Can you work these out from the model? Positions are in its coordinate system, mm. A direction names the side the tool comes from. Round coordinates to 2 decimals unless told otherwise and drop trailing zeros. Write each loop counter-clockwise with the first axis right and the second up, starting at its lowest first coordinate (ties: lowest second). Pieces come first, ordered by that corner, then holes. Notation, with made-up numbers: (60, -26.5) - (73, -26.5) arc R27 ccw to (73, -5.5) - close; hole circle Ø11 at (-31.5, 24). An arc over 180 degrees is marked (long way). One line per item, written item: value. Start each with the question number.
(1) I'm going to push flat-ended pins straight in: pin 1 Ø4 at (x, z) = (21.5, -6.5) entering from -Y; pin 2 Ø8 at (y, z) = (-39, -13) entering from -X; pin 3 Ø5 at (y, z) = (-66, -8.5) entering from -X; pin 4 Ø23 at (x, y) = (0, 115.25) entering from +Z. Where does each tip first touch, or does it pass through?
(2) Thinking about a two-plate mould opening in Y: for faces 1 (the face through (64, -64, -20)), 2 (the face through (-1, 17, -12)), 3 (the face through (-32.08, -144.48, -9.86)), which applies, +Y half, -Y half, draft (parallel to the pull), parting line (faces both ways), or undercut?
(3) I want a section at A-A on y = 0. List the corners of the cut face in (x, z) for me.
(4) I want a section at C-C on x = -105. List the corners of the cut face in (y, z) for me, plus the area to 3 significant figures.
(5) On a 3-axis mill with a long thin cutter (end or side, diameter ignored), from which of +Z, -Z, +X, -X, +Y, -Y can I reach the whole of each face in a straight line? I mean faces 4 (the face through (-17.88, 80.54, -16.06)), 5 (the face through (-2, -31, 0)). Say none if no direction works.
(6) I want a section at D-D on z = -16. List the corners of the cut face in (x, y) for me (3 decimals), plus the area to 3 significant figures.
(7) I want a section at B-B on x = 0. List the corners of the cut face in (y, z) for me, plus the area to 3 significant figures.
(8) If I drill on L1, parallel to Y at x = 0, z = -14; L2, parallel to X at y = 60, z = -6; L3, parallel to Y at x = 113.5, z = -12.25, over which ranges is the centre line in solid material (lowest first)? Write a range as from..to.
from build123d import *

# Parameters (mm, degrees)
F0_R     = 148
F0_R_2   = 8.95
F1_DEPTH = 20
F2_R     = 82.5
F2_R_2   = 8.95
F3_DEPTH = 8
F2_R_3   = 19.05
F4_DEPTH = 20


with BuildPart() as f1:
    # F0 (on Top) → F1 (new body)
    with BuildSketch(Plane.XY):
        Circle(F0_R)
        Circle(F0_R_2, mode=Mode.SUBTRACT)
    extrude(amount=-F1_DEPTH)

    # F2 (on face) → F3 (cut)
    with BuildSketch(Plane(origin=(0, 0, -20), x_dir=(1, 0, 0), z_dir=(0, 0, -1))):
        Circle(F2_R)
        Circle(F2_R_2, mode=Mode.SUBTRACT)
    extrude(amount=-F3_DEPTH, mode=Mode.SUBTRACT)

    # F2 (on face) → F4 (cut, through all)
    with BuildSketch(Plane(origin=(0, 0, -20), x_dir=(1, 0, 0), z_dir=(0, 0, -1))):
        with Locations((-99.809428, 57.625)):
            Circle(F2_R_3)
        with Locations((-99.809428, -57.625)):
            Circle(F2_R_3)
        with Locations((0, -115.25)):
            Circle(F2_R_3)
        with Locations((99.809428, -57.625)):
            Circle(F2_R_3)
        with Locations((99.809428, 57.625)):
            Circle(F2_R_3)
        with Locations((0, 115.25)):
            Circle(F2_R_3)
    extrude(amount=-F4_DEPTH, mode=Mode.SUBTRACT)


with BuildPart() as f5_1:
    # F5: copy of F1
    add(f1.part)


solid = f1.part
Established:
1. pin 1: y = -146.71
1. pin 2: x = -143.8
1. pin 3: x = -133.69
1. pin 4: through
2. face 1: draft
2. face 2: undercut
2. face 3: parting line
3. outline: (-148, -20) - (-82.5, -20) - (-82.5, -12) - (-8.95, -12) - (-8.95, 0) - (-148, 0) - close; (8.95, -12) - (82.5, -12) - (82.5, -20) - (148, -20) - (148, 0) - (8.95, 0) - close
4. outline: (-104.3, -20) - (-75.95, -20) - (-75.95, 0) - (-104.3, 0) - close; (-39.3, -20) - (39.3, -20) - (39.3, 0) - (-39.3, 0) - close; (75.95, -20) - (104.3, -20) - (104.3, 0) - (75.95, 0) - close
4. area: 2,710 mm2
5. face 4: -Z
5. face 5: +Z, +X, -X, +Y, -Y
6. outline: circle Ø296 at (0, 0); hole circle Ø38.1 at (-99.809, -57.625); hole circle Ø38.1 at (-99.809, 57.625); hole circle Ø165 at (0, 0); hole circle Ø38.1 at (0, -115.25); hole circle Ø38.1 at (0, 115.25); hole circle Ø38.1 at (99.809, -57.625); hole circle Ø38.1 at (99.809, 57.625)
6. area: 40,600 mm2
7. outline: (-148, -20) - (-134.3, -20) - (-134.3, 0) - (-148, 0) - close; (-96.2, -20) - (-82.5, -20) - (-82.5, -12) - (-8.95, -12) - (-8.95, 0) - (-96.2, 0) - close; (8.95, -12) - (82.5, -12) - (82.5, -20) - (96.2, -20) - (96.2, 0) - (8.95, 0) - close; (134.3, -20) - (148, -20) - (148, 0) - (134.3, 0) - close
7. area: 2,860 mm2
8. L1: -148..-134.3, -96.2..-82.5, 82.5..96.2, 134.3..148
8. L2: -135.29..-118.71, -80.91..80.91, 118.71..135.29
8. L3: -94.98..-70.87, -44.38..44.38, 70.87..94.98
